Input: part model. Units: mm. Frame: model coordinates. Coordinates: 2 decimals unless noted, no trailing zeros. Order: outer loops, then holes, each group sorted by start corner. A loop starts at its lowest first (then second) coordinate and runs counter-clockwise, first axis right, second up. Notation, with made-up numbers: (23.5, 54) - (33.5, 54) arc R27 cw to (33.5, 76) - close; hole circle Ø1 at (-22.75, -3). An arc over 180 degrees is marked (long way). Use a Markdown table: item, result. Add a question column.
from build123d import *

# Parameters (mm, degrees)
BOSS_EXTRUDE1_DEPTH = 31.2
FILLET1_R           = 1
FILLET2_R           = 1
FILLET3_R           = 1
FILLET4_R           = 1
FILLET20_R          = 1
FILLET21_R          = 1
FILLET22_R          = 1
FILLET23_R          = 1


with BuildPart() as part:
    # Sketch1 → Boss-Extrude1 (new body)
    with BuildSketch(Plane(origin=(0, 0, 0), x_dir=(1, 0, 0), z_dir=(0, 1, 0))):
        with BuildLine():
            Line((-0.8, -0.8), (-0.8, -2.102974084))
            ThreePointArc((-0.8, -2.102974084), (0, -2.25), (0.8, -2.102974084))
            Line((0.8, -2.102974084), (0.8, -0.8))
            Line((0.8, -0.8), (2.102974084, -0.8))
            ThreePointArc((2.102974084, -0.8), (2.25, 0), (2.102974084, 0.8))
            Line((2.102974084, 0.8), (0.8, 0.8))
            Line((0.8, 0.8), (0.8, 2.102974084))
            ThreePointArc((0.8, 2.102974084), (0, 2.25), (-0.8, 2.102974084))
            Line((-0.8, 2.102974084), (-0.8, 0.8))
            Line((-0.8, 0.8), (-2.102974084, 0.8))
            ThreePointArc((-2.102974084, 0.8), (-2.25, 0), (-2.102974084, -0.8))
            Line((-2.102974084, -0.8), (-0.8, -0.8))
        make_face()
    extrude(amount=BOSS_EXTRUDE1_DEPTH)

    # Fillet1
    fillet1_edges = [part.edges().sort_by_distance(p)[0] for p in [
        (-2.25, 0, 0),
    ]]
    fillet(fillet1_edges, radius=FILLET1_R)

    # Fillet2
    fillet2_edges = [part.edges().sort_by_distance(p)[0] for p in [
        (0, 0, 2.25),
    ]]
    fillet(fillet2_edges, radius=FILLET2_R)

    # Fillet3
    fillet3_edges = [part.edges().sort_by_distance(p)[0] for p in [
        (2.25, 0, 0),
    ]]
    fillet(fillet3_edges, radius=FILLET3_R)

    # Fillet4
    fillet4_edges = [part.edges().sort_by_distance(p)[0] for p in [
        (0, 0, -2.25),
    ]]
    fillet(fillet4_edges, radius=FILLET4_R)

    # Fillet20
    fillet20_edges = [part.edges().sort_by_distance(p)[0] for p in [
        (2.25, 31.2, 0),
    ]]
    fillet(fillet20_edges, radius=FILLET20_R)

    # Fillet21
    fillet21_edges = [part.edges().sort_by_distance(p)[0] for p in [
        (0, 31.2, 2.25),
    ]]
    fillet(fillet21_edges, radius=FILLET21_R)

    # Fillet22
    fillet22_edges = [part.edges().sort_by_distance(p)[0] for p in [
        (-2.25, 31.2, 0),
    ]]
    fillet(fillet22_edges, radius=FILLET22_R)

    # Fillet23
    fillet23_edges = [part.edges().sort_by_distance(p)[0] for p in [
        (0, 31.2, -2.25),
    ]]
    fillet(fillet23_edges, radius=FILLET23_R)


solid = part.part
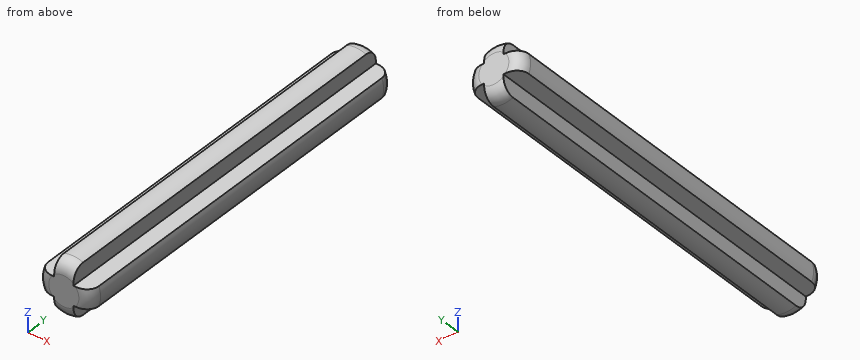
1) Contact query for flat-ended pins moving along their axis: P1, Ø0.7, axis at x = -1, y = 22.5, coming from the -Z side; P2, Ø0.7, axis at x = 1.5, y = 18, coming from the -Z side; P3, Ø1.5, axis at y = 15.5, z = 1, coming from the -X side. Output: stop coordinate, or through.
2) Material intervals for L1, parallel to Z at x = 0.1, y = 25; L2, parallel to Z at x = -1.7, y = 10, sorted ascending.
3) Cut plane A-A (y = 4.5). Return the cut outline in (x, z), and give its area (3 significant figures).
Computed:
| question | item | result |
|---|---|---|
| 1 | P1 | stops at z = -2.15 |
| 1 | P2 | stops at z = -0.8 |
| 1 | P3 | stops at x = -2.24 |
| 2 | L1 | z = -2.25 to 2.25 |
| 2 | L2 | z = -0.8 to 0.8 |
| 3 | outline | (-2.1, -0.8) - (-0.8, -0.8) - (-0.8, -2.1) arc R2.25 ccw to (0.8, -2.1) - (0.8, -0.8) - (2.1, -0.8) arc R2.25 ccw to (2.1, 0.8) - (0.8, 0.8) - (0.8, 2.1) arc R2.25 ccw to (-0.8, 2.1) - (-0.8, 0.8) - (-2.1, 0.8) arc R2.25 ccw to start |
| 3 | area | 11.5 mm2 |
